```python
from build123d import *

# Parameters (mm, degrees)
SKETCH1_W           = 160
SKETCH1_H           = 180
SKETCH1_R           = 75.125
SKETCH1_R_2         = 2.125
BOSS_EXTRUDE1_DEPTH = 12.825
FILLET1_R           = 3


with BuildPart() as part:
    # Sketch1 → Boss-Extrude1 (new body)
    with BuildSketch(Plane(origin=(0, 0, 0), x_dir=(1, 0, 0), z_dir=(0, 1, 0))):
        Rectangle(SKETCH1_W, SKETCH1_H)
        with Locations(Location((0, 0, 0), (0, 0, 270))):
            Circle(SKETCH1_R, mode=Mode.SUBTRACT)
        with Locations(Location((-74, -84, 0), (0, 0, 270))):
            Circle(SKETCH1_R_2, mode=Mode.SUBTRACT)
        with Locations(Location((-74, -42, 0), (0, 0, 270))):
            Circle(SKETCH1_R_2, mode=Mode.SUBTRACT)
        with Locations(Location((-74, 84, 0), (0, 0, 90))):
            Circle(SKETCH1_R_2, mode=Mode.SUBTRACT)
        with Locations(Location((74, -84, 0), (0, 0, 90))):
            Circle(SKETCH1_R_2, mode=Mode.SUBTRACT)
        with Locations(Location((74, -42, 0), (0, 0, 90))):
            Circle(SKETCH1_R_2, mode=Mode.SUBTRACT)
        with Locations(Location((74, 84, 0), (0, 0, 270))):
            Circle(SKETCH1_R_2, mode=Mode.SUBTRACT)
        with Locations(Location((0, -84, 0), (0, 0, 270))):
            Circle(SKETCH1_R_2, mode=Mode.SUBTRACT)
        with Locations(Location((0, 84, 0), (0, 0, 90))):
            Circle(SKETCH1_R_2, mode=Mode.SUBTRACT)
        with Locations(Location((74, 42, 0), (0, 0, 270))):
            Circle(SKETCH1_R_2, mode=Mode.SUBTRACT)
        with Locations(Location((-74, 42, 0), (0, 0, 90))):
            Circle(SKETCH1_R_2, mode=Mode.SUBTRACT)
    extrude(amount=BOSS_EXTRUDE1_DEPTH)

    # Fillet1
    fillet1_edges = [part.edges().sort_by_distance(p)[0] for p in [
        (80, 6.4125, 90),
        (-80, 6.4125, 90),
        (-80, 6.4125, -90),
        (80, 6.4125, -90),
    ]]
    fillet(fillet1_edges, radius=FILLET1_R)


solid = part.part
```
CAD build for the part. Positions are in the model's coordinates, mm. Round coordinates to 2 decimals unless told otherwise and drop trailing zeros. Write each loop counter-clockwise with the first axis right and the second up, starting at its lowest first coordinate (ties: lowest second). Pieces come first, ordered by that corner, then holes.
Item 1: Band-saw the part on C-C on y = 7.75. Give the number of separate pieces and of enclosed holes in the cut face, then the cut area to 3 significant figures.
Filled in:
separate pieces: 1
enclosed holes: 11
area: 10,900 mm2
Item 2: Mould opens along X. For faces 1 (the cylindrical face through (76.107, 6.323, -42.277)), 2 (the flat face through (-1, 6, -90)), 3 (the flat face through (80, 6, 1)), 4 (the cylindrical face through (-71.893, 6.323, 41.723)) say: released by +X, released by -X, zero draft, split by the parting line, or undercut.
Filled in:
face 1: undercut
face 2: zero draft
face 3: released by +X
face 4: undercut
Item 3: Band-saw the part on B-B on z = 0. Write the cut outline in (x, y) (3 decimals).
Filled in:
outline: (-80, 0) - (-75.125, 0) - (-75.125, 12.825) - (-80, 12.825) - close; (75.125, 0) - (80, 0) - (80, 12.825) - (75.125, 12.825) - close
Item 4: Band-saw the part on A-A on x = 0. Write the cut outline in (y, z) (3 decimals).
Filled in:
outline: (0, -90) - (12.825, -90) - (12.825, -86.125) - (0, -86.125) - close; (0, -81.875) - (12.825, -81.875) - (12.825, -75.125) - (0, -75.125) - close; (0, 75.125) - (12.825, 75.125) - (12.825, 81.875) - (0, 81.875) - close; (0, 86.125) - (12.825, 86.125) - (12.825, 90) - (0, 90) - close
Item 5: Band-saw the part on D-D on z = -84. Write the cut outline in (x, y) (3 decimals), then the cut area to 3 significant figures.
Filled in:
outline: (-80, 0) - (-76.125, 0) - (-76.125, 12.825) - (-80, 12.825) - close; (-71.875, 0) - (-2.125, 0) - (-2.125, 12.825) - (-71.875, 12.825) - close; (2.125, 0) - (71.875, 0) - (71.875, 12.825) - (2.125, 12.825) - close; (76.125, 0) - (80, 0) - (80, 12.825) - (76.125, 12.825) - close
area: 1,890 mm2
Item 6: Drill centre lines: L1, parallel to X at y = 6.5, z = 84 (3 decimals); L2, parallel to X at y = 6.75, z = -41.5; L3, parallel to X at y = 1, z = -34. Where is each one in solid material? Low to high.
Filled in:
L1: x = -80 to -76.125, -71.875 to -2.125, 2.125 to 71.875, 76.125 to 80
L2: x = -80 to -76.07, -71.93 to -62.62, 62.62 to 71.93, 76.07 to 80
L3: x = -80 to -66.99, 66.99 to 80
